Input: part model. Units: mm. Frame: model coordinates. Face numbers are marked on the shaded views. Give positions to 0.01 mm unless a question says otherwise; leave off trailing zeros. Loops run counter-clockwise (first coordinate to the right, second up) from the corner with the lowest first, then second, coordinate; pieces in that order, holes last. Notation, with made-up numbers: (-9, 26.5) - (42, 26.5) arc R24 cw to (42, 43.5) - close; hole circle Ø9 at (42, 67.5). An arc over 180 degrees is marked (long way). Answer as a JSON object with one key per item and string values. Group by question number.
(1) Mould query, pull axis Y, two halves, no side actions, for the marked faces 1, 2 and 3. Classes: +Y half, -Y half, draft (parallel to the pull), parting line (faces both ways), or undercut.
(2) Material intervals for L1, parallel to Y at x = -7, z = 0.4; L2, parallel to Y at x = -8, z = 2.1; L3, parallel to Y at x = -0.75, z = 1, sorted ascending.
(3) Section query B-B (z = 4.2). Return loops of the section in (x, y), plus the area to 3 significant figures.
(4) Pin query (flat end, axial travel): P1, Ø1.5, axis at x = -1.5, z = 4, coming from the +Y side. Return the tip coordinate at first contact, or that it passes through.
(5) Section query A-A (y = 10). Return loops of the section in (x, z).
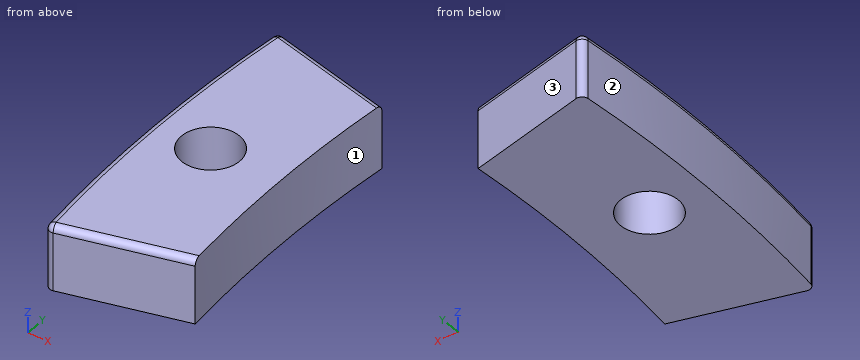
```python
from build123d import *

# Parameters (mm, degrees)
F1_DEPTH = 5
F2_R     = 2.25
F3_DEPTH = 25
F4_R     = 0.5


with BuildPart() as f1:
    # F0 (on Top) → F1 (new body)
    with BuildSketch(Plane.XY):
        with BuildLine():
            ThreePointArc((-9.788721, 22.5), (-10.501256, 10), (-9.788721, -2.5))
            Line((-9.788721, -2.5), (0, 0))
            ThreePointArc((0, 0), (-0.501256, 10), (0, 20))
            Line((0, 20), (-9.788721, 22.5))
        make_face()
    extrude(amount=F1_DEPTH)

    # F2 (on face) → F3 (cut)
    with BuildSketch(Plane.XY.offset(5)):
        with Locations((-6.001256, 10)):
            Circle(F2_R)
    extrude(amount=-F3_DEPTH, mode=Mode.SUBTRACT)

    # F4
    f4_edges = [f1.edges().sort_by_distance(p)[0] for p in [
        (-4.894361, -1.25, 5),
        (-9.788721, -2.5, 2.5),
        (-10.501256, 10, 5),
        (-9.788721, 22.5, 2.5),
        (-4.894361, 21.25, 5),
    ]]
    fillet(f4_edges, radius=F4_R)


solid = f1.part
```
Recorded:
{
 "1": {"face 1": "undercut", "face 2": "parting line", "face 3": "+Y half"},
 "2": {"L1": "y = -1.79 to 7.98, 12.02 to 21.79", "L2": "y = -2.04 to 8.97, 11.03 to 22.04", "L3": "y = -0.19 to 20.19"},
 "3": {"outline": "(-9.85, -1.93) arc R0.5 ccw to (-9.23, -2.36) - (0, 0) arc R100 cw to (0, 20) - (-9.23, 22.36) arc R0.5 ccw to (-9.85, 21.93) arc R110 ccw to start; hole circle Ø4.5 at (-6, 10)", "area": "209 mm^2"},
 "4": {"P1": "stops at y = 20.57"},
 "5": {"outline": "(-10.5, 0) - (-8.25, 0) - (-8.25, 5) - (-10, 5) arc R0.5 ccw to (-10.5, 4.5) - close; (-3.75, 0) - (-0.5, 0) - (-0.5, 5) - (-3.75, 5) - close"}
}
